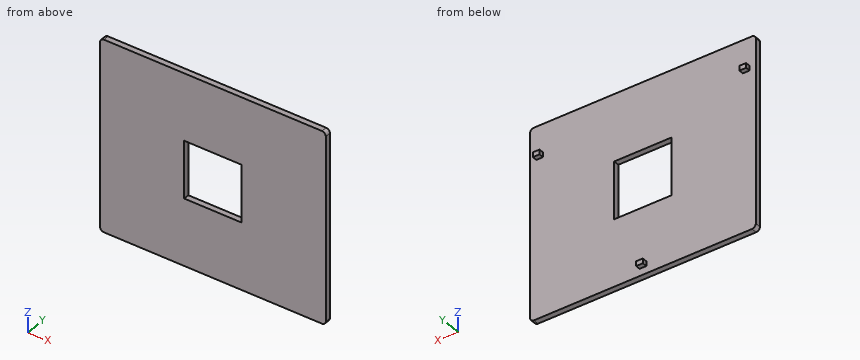
from build123d import *

# Parameters (mm, degrees)
SKETCH1_W           = 118
SKETCH1_H           = 100
SKETCH1_W_2         = 30
SKETCH1_H_2         = 30
BOSS_EXTRUDE1_DEPTH = 3
SKETCH2_W           = 3.5
SKETCH2_H           = 2.5
BOSS_EXTRUDE2_DEPTH = 2.5
FILLET1_R           = 2


with BuildPart() as part:
    # Sketch1 → Boss-Extrude1 (new body)
    with BuildSketch(Plane(origin=(0, 0, 0), x_dir=(1, 0, 0), z_dir=(0, 1, 0))):
        Rectangle(SKETCH1_W, SKETCH1_H)
        Rectangle(SKETCH1_W_2, SKETCH1_H_2, mode=Mode.SUBTRACT)
    extrude(amount=BOSS_EXTRUDE1_DEPTH)

    # Sketch2 → Boss-Extrude2 (add)
    with BuildSketch(Plane(origin=(0, 3, 0), x_dir=(1, 0, 0), z_dir=(0, 1, 0))):
        with Locations((54, -34)):
            Rectangle(SKETCH2_W, SKETCH2_H)
        with Locations((-54, -34)):
            Rectangle(SKETCH2_W, SKETCH2_H)
        with Locations((0, 45)):
            Rectangle(SKETCH2_W, SKETCH2_H)
    extrude(amount=BOSS_EXTRUDE2_DEPTH)

    # Fillet1
    fillet1_edges = [part.edges().sort_by_distance(p)[0] for p in [
        (59, 1.5, 50),
        (-59, 1.5, 50),
        (-59, 1.5, -50),
        (59, 1.5, -50),
    ]]
    fillet(fillet1_edges, radius=FILLET1_R)


solid = part.part
CAD build for the part. Positions are in the model's coordinates, mm. Give positions to 0.01 mm unless a question says otherwise; leave off trailing zeros. Loops run counter-clockwise (first coordinate to the right, second up) from the corner with the lowest first, then second, coordinate; pieces in that order, holes last. Notation, with made-up numbers: M 71,4 L 120,4 A22 ccw 120,21 Z; hole C 55,-24 d2. An arc over 180 degrees is marked long. Answer in a Markdown table with one row per item. Add a question column.
Item 1: Probe probe 1 along Z at (x, y) = (1, 1.35); probe 2 along X at (y, z) = (0.75, -3.5); probe 3 along Y at (x, z) = (-51.5, 0.5). List the from-to ranges inside material, lowest first.
Item 2: Band-saw the part on B-B on x = -6.5. Give the cut face in (y, z).
Item 3: Band-saw the part on C-C on y = 3.9. Give the cut face in (x, z).
Item 4: Band-saw the part on A-A on z = 7.5. Give the cut face in (x, y), then the cut area to 3 significant figures.
Item 5: Band-saw the part on D-D on x = -23.5. Give the cut face in (y, z), then the cut area to 3 significant figures.
Item 6: Drop flat-ended pins along their axis: P1, Ø10, axis at x = 20, z = 39, coming from the +Y side; P2, Ø1.2, axis at x = 54, y = 4, coming from the +Z side; P3, Ø1.2, axis at y = 4, z = -45, coming from the +X side. Give the stop position or say it passes through.
Reply:
| question | item | result |
|---|---|---|
| 1 | probe 1 | z = -50 to -15, 15 to 50 |
| 1 | probe 2 | x = -59 to -15, 15 to 59 |
| 1 | probe 3 | y = 0 to 3 |
| 2 | outline | M 0,-50 L 3,-50 L 3,-15 L 0,-15 Z; M 0,15 L 3,15 L 3,50 L 0,50 Z |
| 3 | outline | M -55.75,32.75 L -52.25,32.75 L -52.25,35.25 L -55.75,35.25 Z; M -1.75,-46.25 L 1.75,-46.25 L 1.75,-43.75 L -1.75,-43.75 Z; M 52.25,32.75 L 55.75,32.75 L 55.75,35.25 L 52.25,35.25 Z |
| 4 | outline | M -59,0 L -15,0 L -15,3 L -59,3 Z; M 15,0 L 59,0 L 59,3 L 15,3 Z |
| 4 | area | 264 mm^2 |
| 5 | outline | M 0,-50 L 3,-50 L 3,50 L 0,50 Z |
| 5 | area | 300 mm^2 |
| 6 | P1 | stops at y = 3 |
| 6 | P2 | stops at z = 35.25 |
| 6 | P3 | stops at x = 1.75 |
